Geometry: final body of the model. Coordinates: model frame, mm. A direction names the side the tool comes from. Coordinates: 2 decimals unless noted, no trailing zeros. Write each loop counter-clockwise with the first axis right and the second up, starting at its lowest first coordinate (ties: lowest second). Pieces come first, ordered by that corner, then holes. Notation, with made-up numbers: (84.25, 14.25) - (133.25, 14.25) arc R9 cw to (133.25, 29.25) - close; hole circle Ø10 at (-10, -36.5). An arc over 180 degrees is marked (long way). Put each result on its own line as item: value.
Autodesk Inventor part; units mm, degrees
ref_plane "YZ Plane" through (0, 0, 0) normal (1, 0, 0) x (0, 1, 0)
ref_plane "XZ Plane" through (0, 0, 0) normal (0, 1, 0) x (-1, 0, 0)
ref_plane "XY Plane" through (0, 0, 0) normal (0, 0, 1) x (1, 0, 0)
sketch "shape" plane through (0, 0, 0) normal (0, 0, 1) x (1, 0, 0)
  line L0 (-18.25, 18.25) -> (18.25, 18.25)
  line L1 (18.25, 18.25) -> (18.25, -18.25)
  line L2 (18.25, -18.25) -> (-18.25, -18.25)
  line L3 (-18.25, -18.25) -> (-18.25, 18.25)
  line L4 (-15.5, 15.5) -> (15.5, 15.5)
  line L5 (15.5, 15.5) -> (15.5, -15.5)
  line L6 (15.5, -15.5) -> (-15.5, -15.5)
  line L7 (-15.5, -15.5) -> (-15.5, 15.5)
  line L8 (9.5, 2.5) -> (15.5, 2.5)
  line L9 (15.5, 2.5) -> (15.5, -2.5)
  line L10 (15.5, -2.5) -> (9.5, -2.5)
  line L11 (9.5, -2.5) -> (9.5, 2.5)
  line L12 (-0.5, 15.5) -> (9.5, 15.5)
  line L13 (9.5, 15.5) -> (9.5, 11.5)
  line L14 (9.5, 11.5) -> (-0.5, 11.5)
  line L15 (-0.5, 11.5) -> (-0.5, 15.5)
  line L16 (-8.5, -11.5) -> (9.5, -11.5)
  line L17 (9.5, -11.5) -> (9.5, -15.5)
  line L18 (9.5, -15.5) -> (-8.5, -15.5)
  line L19 (-8.5, -15.5) -> (-8.5, -11.5)
  line L20 (-15.5, 0) -> (-8.5, 0)
  line L21 (-8.5, 0) -> (-8.5, -2.5)
  line L22 (-8.5, -2.5) -> (-15.5, -2.5)
  line L23 (-15.5, -2.5) -> (-15.5, 0)
  circle A0 centre (-9, 9) radius 8.5
  line L24 (-3, 24.25) -> (3, 24.25)
  line L25 (3, 24.25) -> (3, 18.25)
  line L26 (3, 18.25) -> (-3, 18.25)
  line L27 (-3, 18.25) -> (-3, 24.25)
  line L28 (-3, -18.25) -> (3, -18.25)
  line L29 (3, -18.25) -> (3, -24.25)
  line L30 (3, -24.25) -> (-3, -24.25)
  line L31 (-3, -24.25) -> (-3, -18.25)
  circle A1 centre (0, -21.25) radius 1.75
  circle A2 centre (0, 21.25) radius 1.75
  point P0 (0, 0)
  point P1 (-18.25, 0)
  point P2 (0, 18.25)
  point P3 (-15.5, 0)
  point P4 (0, 15.5)
  point P5 (0, 24.25)
  point P6 (3, 21.25)
  point P7 (0, -24.25)
  point P8 (3, -21.25)
  dimension "d1" = 36.5
  dimension "d2" = 31
  dimension "d3" = 31
  dimension "d4" = 5
  dimension "d5" = 6
  dimension "d6" = 13
  dimension "d7" = 10
  dimension "d8" = 4
  dimension "d9" = 6
  dimension "d10" = 18
  dimension "d11" = 4
  dimension "d12" = 6
  dimension "d13" = 7
  dimension "d14" = 2.5
  dimension "d15" = 13
  dimension "d16" = 17
  dimension "d17" = 6.5
  dimension "d18" = 6.5
  dimension "d21" = 6
  dimension "d23" = 3.5
extrude "over pcb" add sketch "shape" along normal blind 1.5 contours L0 L1 L2 L3 | L27 L24 L25 L0 | L2 L29 L30 L31 | L4 L13 L14 L15 | L5 L10 L11 L8 | L20 L21 L22 L7 | L6 L19 L16 L17
extrude "around pcb" add sketch "shape" against normal blind 1.5
equation "\"d18\" = d17"
properties part number "MCP73871_holder"
1. Mould query, pull axis X, two halves, no side actions, for faces 6 (the flat face through (9.5, -13, 1)), 7 (the flat face through (-11, 18.25, 0)), 8 (the flat face through (-3, 21, 0)). Classes: +X half, -X half, draft (parallel to the pull), parting line (faces both ways), or undercut.
Answer below:
face 6: undercut
face 7: draft
face 8: -X half
2. Section query D-D (y = 12). Return loops of the section in (x, z), then the cut area to 3 significant figures.
Answer below:
outline: (-18.25, -1.5) - (-16.95, -1.5) - (-16.95, 1.5) - (-18.25, 1.5) - close; (-0.5, 0) - (9.5, 0) - (9.5, 1.5) - (-0.5, 1.5) - close; (15.5, -1.5) - (18.25, -1.5) - (18.25, 1.5) - (15.5, 1.5) - close
area: 27.1 mm²
3. Set-up query: faces 1 (the flat face through (-11, -18.25, 0)), 2 (the flat face through (3, -21, 0)), 3 (the flat face through (-18.25, 0, 0)), 4 (the flat face through (0, -11.5, 1)), 5 (the flat face through (5.9, 15.5, -0.4)). Return all of +Z, -Z, +X, -X, +Y, -Y with unobstructed straight access to the full face (end or side cutting, diameter ignored); none if empty.
Answer below:
face 1: +Z, -Z, -X, -Y
face 2: +Z, -Z, +X, -Y
face 3: +Z, -Z, -X, +Y, -Y
face 4: +Z, -Z
face 5: -Z
4. Section query C-C (x = 9). Return loops of the section in (y, z), then the cut area to 3 significant figures.
Answer below:
outline: (-18.25, -1.5) - (-15.5, -1.5) - (-15.5, 0) - (-11.5, 0) - (-11.5, 1.5) - (-18.25, 1.5) - close; (11.5, 0) - (15.5, 0) - (15.5, -1.5) - (18.25, -1.5) - (18.25, 1.5) - (11.5, 1.5) - close
area: 28.5 mm²
5. Pin query (flat end, axial travel): pin 1 Ø0.8 at (x, y) = (-11, -1) entering from -Z; pin 2 Ø1 at (x, y) = (14.5, 11.5) entering from +Z; pin 3 Ø1.6 at (x, z) = (-13.5, 1) entering from +Y; pin 4 Ø1.5 at (y, z) = (-20.5, -0.5) entering from +X. Return the tip coordinate at first contact, or that it passes through.
Answer below:
pin 1: stops at z = 0
pin 2: passes through
pin 3: stops at y = 18.25
pin 4: stops at x = 3
6. Section query B-B (x = 0). Return loops of the section in (y, z).
Answer below:
outline: (-24.25, -1.5) - (-23, -1.5) - (-23, 1.5) - (-24.25, 1.5) - close; (-19.5, -1.5) - (-15.5, -1.5) - (-15.5, 0) - (-11.5, 0) - (-11.5, 1.5) - (-19.5, 1.5) - close; (11.5, 0) - (15.5, 0) - (15.5, -1.5) - (19.5, -1.5) - (19.5, 1.5) - (11.5, 1.5) - close; (23, -1.5) - (24.25, -1.5) - (24.25, 1.5) - (23, 1.5) - close
7. Section query A-A (y = 21.25). Return loops of the section in (x, z).
Answer below:
outline: (-3, -1.5) - (-1.75, -1.5) - (-1.75, 1.5) - (-3, 1.5) - close; (1.75, -1.5) - (3, -1.5) - (3, 1.5) - (1.75, 1.5) - close
8. Ray query, probe 1 along Y at (x, z) = (0, 0.55); probe 2 along Y at (x, z) = (10.5, 1); probe 3 along X at (y, z) = (-1, 0.15). Return the intervals inside material, ascending. Write a range as from..to.
Answer below:
probe 1: y = -24.25..-23, -19.5..-11.5, 11.5..19.5, 23..24.25
probe 2: y = -18.25..-15.5, -2.5..2.5, 15.5..18.25
probe 3: x = -18.25..-8.5, 9.5..18.25
